Autodesk Inventor part; units mm, degrees
ref_plane "YZ Plane" through (0, 0, 0) normal (1, 0, 0) x (0, 1, 0)
ref_plane "XZ Plane" through (0, 0, 0) normal (0, 1, 0) x (-1, 0, 0)
ref_plane "XY Plane" through (0, 0, 0) normal (0, 0, 1) x (1, 0, 0)
sketch "Sketch1" plane through (0, 0, 0) normal (0, 1, 0) x (-1, 0, 0)
  arc A0 (-8.2614, -8) -> (-8.2614, 8) centre (0, 0) ccw
  line L0 (-9.6047, 8) -> (-8.2614, 8)
  arc A1 (-9.6047, 8) -> (-9.6047, -8) centre (0, 0) ccw
  line L1 (-8.2614, -8) -> (-9.6047, -8)
extrude "Extrusion1" add sketch "Sketch1" along normal blind 3
sketch "Sketch2" plane through (0, 0, 0) normal (0, 0, 1) x (1, 0, 0)
  line L0 (12.9833, 2.607) -> (12.9833, 0)
  line L1 (12.9833, 0) -> (-11.5556, 0)
  line L2 (-11.5556, 0) -> (12.9833, 2)
  point P0 (0, 0)
extrude "Extrusion2" cut sketch "Sketch2" along normal mid plane 26.25
sketch "Sketch3" plane through (0, 3, 0) normal (0, 1, 0) x (1, 0, 0)
  line L0 (9.6047, 8) -> (8.2614, 8)
  arc A0 (8.2614, 8) -> (8.2614, -8) centre (0, 0) ccw
  line L1 (8.2614, -8) -> (9.6047, -8)
  arc A1 (9.6047, -8) -> (9.6047, 8) centre (0, 0) ccw
extrude "Extrusion3" cut sketch "Sketch3" against normal blind 0.75
properties part number "5_grader_adapter" material "S355J2+N"
CAD build for the part. Positions are in the model's coordinates, mm. Give positions to 0.01 mm unless a question says otherwise; leave off trailing zeros. Loops run counter-clockwise (first coordinate to the right, second up) from the corner with the lowest first, then second, coordinate; pieces in that order, holes last. Notation, with made-up numbers: M 77,57.25 L 94,57.25 A17 ccw 94,63.25 Z; hole C 49,55.25 d5. An arc over 180 degrees is marked long. One line per question, with ' | ' between items. Start each with the question number.
1. Flat gauge pins, fed straight in: pin 1 (1 mm diameter, centred on y = 1, z = -2.5, fed in from -X); pin 2 (0.5 mm diameter, centred on x = 9, y = 2, fed in from -Z); pin 3 (0.5 mm diameter, centred on x = 9, y = 2, fed in from +Z). Where does each tip first touch, or does it go through?
2. Saw through at A-A on y = 1. Give the cut face in (x, z), plus the area to 3 significant figures.
3. Saw through at C-C on x = 0. Give the cut face in (y, z), plus the area to 3 significant figures.
4. Probe L1, parallel to Z at x = 8.75, y = 2.15; L2, parallel to X at y = 2.15, z = 0.25; L3, parallel to Y at x = -3.5, z = 7.75. List the from-to ranges inside material, lowest first. Write a range as from..to.
5. Saw through at B-B on z = 0. Give the cut face in (x, y).
Result sheet:
1) pin 1: stops at x = -11.32 | pin 2: stops at z = -8 | pin 3: stops at z = 8
2) outline: M 0.71,-11.48 L 0.71,11.48 A11.5 ccw long Z | area: 224 mm^2
3) outline: M 0.94,-11.5 L 2.25,-11.5 L 2.25,11.5 L 0.94,11.5 Z | area: 30.1 mm^2
4) L1: z = -8..8 | L2: x = -11.5..12.5 | L3: y = 0.66..2.25
5) outline: M -11.5,0 L 12.5,1.96 L 12.5,2.25 L -11.5,2.25 Z
